Work out the finished part from the listing and answer in its coordinate system (mm). Round coordinates to 2 decimals unless told otherwise and drop trailing zeros. Write each loop counter-clockwise with the first axis right and the second up, starting at its lowest first coordinate (ties: lowest second). Pieces come first, ordered by that corner, then holes.
1. Find section B-B (x = 145). Write down the section's boundary in (y, z), and give its area (3 significant figures).
2. Find section A-A (y = 15). Write down the section's boundary in (x, z).
3. Straight lines are drawn through the part: probe 1 along Y at (x, z) = (125, 4.25); probe 2 along Y at (x, z) = (146, 8); probe 3 along X at (y, z) = (143.5, 5). For each, find the intervals that lie inside material, in ascending order.
4. Find section D-D (z = 8.5). Write down the section's boundary in (x, y), and give its area (3 significant figures).
Autodesk Inventor part; units mm, degrees
ref_plane "YZ Plane" through (0, 0, 0) normal (1, 0, 0) x (0, 1, 0)
ref_plane "XZ Plane" through (0, 0, 0) normal (0, 1, 0) x (-1, 0, 0)
ref_plane "XY Plane" through (0, 0, 0) normal (0, 0, 1) x (1, 0, 0)
sketch "Sketch1" plane through (0, 0, 0) normal (0, 0, 1) x (1, 0, 0)
  line L0 (0, 0) -> (160, 0)
  line L1 (160, 0) -> (160, 160)
  line L2 (160, 160) -> (0, 160)
  line L3 (0, 160) -> (0, 0)
  dimension "d0" = 160
  dimension "d1" = 160
extrude "Extrusion1" add sketch "Sketch1" along normal blind 10
sketch "Sketch2" plane through (0, 0, 10) normal (0, 0, 1) x (1, 0, 0)
  line L0 (0, 0) -> (160, 0)
  line L1 (0, 0) -> (15, 0)
  line L2 (15, 0) -> (15, 15)
  line L3 (160, 160) -> (0, 160)
  line L4 (0, 160) -> (15, 160)
  line L5 (15, 160) -> (15, 145)
  line L6 (160, 0) -> (160, 160)
  line L7 (160, 160) -> (145, 160)
  line L8 (145, 160) -> (145, 143.5)
  line L9 (160, 0) -> (160, 15)
  line L10 (160, 15) -> (145, 15)
  circle A0 centre (15, 145) radius 7.5
  circle A1 centre (145, 143.5) radius 7.5
  circle A2 centre (145, 15) radius 7.5
  circle A3 centre (15, 15) radius 7.5
  dimension "d4" = 15
  dimension "d5" = 15
  dimension "d6" = 15
  dimension "d7" = 15
  dimension "d8" = 15
  dimension "d9" = 16.5
  dimension "d10" = 15
  dimension "d11" = 15
  dimension "d12" = 15
  dimension "d13" = 15
  dimension "d14" = 15
  dimension "d15" = 15
extrude "Extrusion2" cut sketch "Sketch2" against normal blind 10
sketch "Sketch3" plane through (0, 0, 10) normal (0, 0, 1) x (1, 0, 0)
  line L0 (0, 160) -> (0, 0)
  line L1 (0, 0) -> (80, 0)
  line L2 (0, 0) -> (160, 0)
  line L3 (80, 0) -> (0, 0)
  line L4 (0, 0) -> (80, 0)
  dimension "d18" = 80
  dimension "d19" = 80
  dimension "d20" = 80
sketch "Sketch4" plane through (0, 0, 10) normal (0, 0, 1) x (1, 0, 0)
  line L0 (0, 0) -> (160, 0)
  line L1 (0, 0) -> (0, 80)
  line L2 (0, 160) -> (0, 0)
  line L3 (0, 80) -> (80, 80)
  line L4 (87.0711, 87.0711) -> (89.6593, 77.4118)
  line L5 (89.6593, 77.4118) -> (82.5882, 70.3407)
  line L6 (82.5882, 70.3407) -> (72.9289, 72.9289)
  line L7 (72.9289, 72.9289) -> (70.3407, 82.5882)
  line L8 (70.3407, 82.5882) -> (77.4118, 89.6593)
  line L9 (77.4118, 89.6593) -> (87.0711, 87.0711)
  line L10 (160, 0) -> (160, 160)
  line L11 (160, 160) -> (160, 80)
  dimension "d21" = 80
  dimension "d22" = 80
  dimension "d23" = 10
  dimension "d24" = 80
sketch "Sketch5" plane through (0, 0, 10) normal (0, 0, 1) x (1, 0, 0)
  line L0 (160, 0) -> (160, 160)
  line L1 (160, 80) -> (125, 80)
  circle A0 centre (125, 80) radius 29
  point P0 (0, 0)
  dimension "d25" = 35
  dimension "d26" = 58
extrude "Extrusion3" cut sketch "Sketch4" against normal blind 10
extrude "Extrusion4" cut sketch "Sketch5" against normal blind 10
properties part number "102"
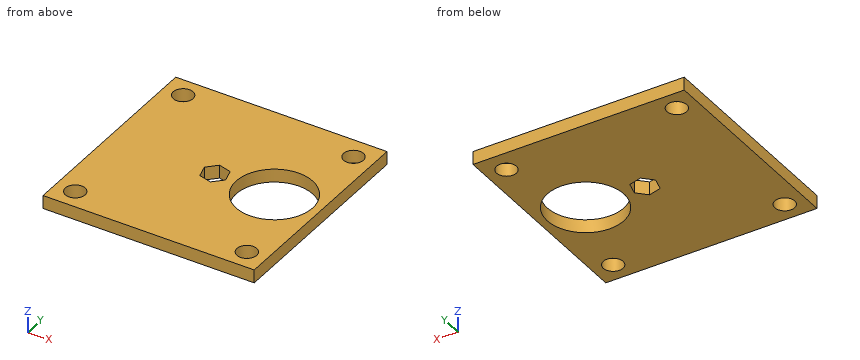
Worked answers:
1. outline: (0, 0) - (7.5, 0) - (7.5, 10) - (0, 10) - close; (22.5, 0) - (59, 0) - (59, 10) - (22.5, 10) - close; (101, 0) - (136, 0) - (136, 10) - (101, 10) - close; (151, 0) - (160, 0) - (160, 10) - (151, 10) - close
1. area: 880 mm2
2. outline: (0, 0) - (7.5, 0) - (7.5, 10) - (0, 10) - close; (22.5, 0) - (137.5, 0) - (137.5, 10) - (22.5, 10) - close; (152.5, 0) - (160, 0) - (160, 10) - (152.5, 10) - close
3. probe 1: y = 0 to 51, 109 to 160
3. probe 2: y = 0 to 7.57, 22.43 to 60, 100 to 136.07, 150.93 to 160
3. probe 3: x = 0 to 7.65, 22.35 to 137.5, 152.5 to 160
4. outline: (0, 0) - (160, 0) - (160, 160) - (0, 160) - close; hole circle Ø15 at (15, 15); hole circle Ø15 at (15, 145); hole (70.34, 82.59) - (72.93, 72.93) - (82.59, 70.34) - (89.66, 77.41) - (87.07, 87.07) - (77.41, 89.66) - close; hole circle Ø58 at (125, 80); hole circle Ø15 at (145, 15); hole circle Ø15 at (145, 143.5)
4. area: 22,000 mm2
